Geometry: final body of the model. Coordinates: model frame, mm. A direction names the side the tool comes from. Give positions to 0.01 mm unless a question says otherwise; leave off trailing zeros. Loops run counter-clockwise (first coordinate to the right, second up) from the corner with the lowest first, then second, coordinate; pieces in that order, holes last.
1. Section B-B, the plane x = 181.5. Output: boundary loops of the cut face in (y, z).
2. Section C-C, the plane z = 21.5. Output: boundary loops of the cut face in (x, y), then the cut area to 3 significant figures.
3. Section A-A, the plane y = 1.4. Output: boundary loops of the cut face in (x, z), then the cut area to 3 significant figures.
4. Material intervals for line 1 along Z through (x, y) = (210.29, 1.4); line 2 along Z through (x, y) = (66, 1.35); line 3 along X through (y, z) = (1.75, 41.08), sorted ascending.
5. Access query for faces 1 (the face through (129, 0, -2)), 2 (the face through (241.4, 2.5, -15.1)). Directions: +Z, -Z, +X, -X, +Y, -Y. A direction counts if a zero-diameter tool reaches every point of the face in a straight line with its end or side. Return the directions, or none.
6. First-contact query: P1, Ø4, axis at x = 210.29, z = -41.08, coming from the +Y side; P2, Ø2.5, axis at x = 121, y = 1.5, coming from the +Z side; P3, Ø1.5, axis at x = 165, y = 1.5, coming from the -Z side. Flat tips, straight axial feed; report the tip coordinate or a pass-through.
7. Draft query along Z for faces 3 (the face through (243.37, 2.465, -79.146)), 4 (the face through (254.323, 2.465, -104.043)), 5 (the face through (254.125, 2.465, 104.241)). Return one class per face: +Z half, -Z half, draft (parallel to the pull), parting line (faces both ways), or undercut.
from build123d import *

# Parameters (mm, degrees)
BOSS_EXTRUDE1_DEPTH = 5
SKETCH2_R           = 2.1
CUT_EXTRUDE1_DEPTH  = 5
SKETCH5_R           = 2.1
CUT_EXTRUDE4_DEPTH  = 10


with BuildPart() as part:
    # Sketch1 → Boss-Extrude1 (new body)
    with BuildSketch(Plane(origin=(0, 0, 0), x_dir=(1, 0, 0), z_dir=(0, 1, 0))):
        Polygon((0, 30), (0, -30), (55.94, -90), (225.94, -90), (247.153203436, -111.213203436), (261.295339059, -97.071067812), (225.94, -61.715728753), (256.965728753, -30.69), (226.32179728, 0), (256.965728753, 30.69), (225.94, 61.715728753), (261.295339059, 97.071067812), (247.153203436, 111.213203436), (225.94, 90), (55.94, 90), align=None)
    extrude(amount=BOSS_EXTRUDE1_DEPTH)

    # Sketch2 → Cut-Extrude1 (cut)
    with BuildSketch(Plane(origin=(0, 5, 0), x_dir=(1, 0, 0), z_dir=(0, 1, 0))):
        with Locations(Location((210.29, 41.08, 0), (0, 0, 270))):
            Circle(SKETCH2_R)
        with Locations(Location((210.29, -41.08, 0), (0, 0, 90))):
            Circle(SKETCH2_R)
    extrude(amount=-CUT_EXTRUDE1_DEPTH, mode=Mode.SUBTRACT)

    # Sketch5 → Cut-Extrude4 (cut)
    with BuildSketch(Plane(origin=(0, 5, 0), x_dir=(1, 0, 0), z_dir=(0, 1, 0))):
        with Locations(Location((67.37, 41.08, 0), (0, 0, 270))):
            Circle(SKETCH5_R)
        with Locations(Location((67.36, -41.08, 0), (0, 0, 270))):
            Circle(SKETCH5_R)
    extrude(amount=-CUT_EXTRUDE4_DEPTH, mode=Mode.SUBTRACT)


solid = part.part
Answers below:
1. outline: (0, -90) - (5, -90) - (5, 90) - (0, 90) - close
2. outline: (0, 0) - (247.79, 0) - (247.79, 5) - (0, 5) - close
2. area: 1,240 mm2
3. outline: (0, -30) - (55.94, -90) - (225.94, -90) - (247.15, -111.21) - (261.3, -97.07) - (225.94, -61.72) - (256.97, -30.69) - (226.32, 0) - (256.97, 30.69) - (225.94, 61.72) - (261.3, 97.07) - (247.15, 111.21) - (225.94, 90) - (55.94, 90) - (0, 30) - close; hole circle Ø4.2 at (67.36, 41.08); hole circle Ø4.2 at (67.37, -41.08); hole circle Ø4.2 at (210.29, -41.08); hole circle Ø4.2 at (210.29, 41.08)
3. area: 40,800 mm2
4. line 1: z = -90 to -43.18, -38.98 to 38.98, 43.18 to 90
4. line 2: z = -90 to -42.67, -39.49 to 39.48, 42.68 to 90
4. line 3: x = 10.33 to 65.26, 69.46 to 208.19, 212.39 to 246.58
5. face 1: +Z, -Z, +X, -X, -Y
5. face 2: +X, +Y, -Y
6. P1: passes through
6. P2: stops at z = 90
6. P3: stops at z = -90
7. face 3: undercut
7. face 4: -Z half
7. face 5: +Z half
